Verification items for the finished model (mm, model axes). A direction names the side the tool comes from. Round coordinates to 2 decimals unless told otherwise and drop trailing zeros. Loops run counter-clockwise (first coordinate to the right, second up) from the corner with the lowest first, then second, coordinate; pieces in that order, holes last.
from build123d import *

# Parameters (mm, degrees)
SKETCH2_W          = 2.5
SKETCH2_H          = 3.5
CUT_EXTRUDE1_DEPTH = 3.5
FILLET1_R          = 0.5
CUT_EXTRUDE2_DEPTH = 0.5


with BuildPart() as part:
    # Sketch1 → Revolve1 (revolve)
    with BuildSketch(Plane.XY, mode=Mode.PRIVATE) as revolve1_sk:
        Polygon((0, 7.25), (5, 7.25), (5, 1.25), (8, 1.25), (8, 0), (0, 0), align=None)
    revolve(revolve1_sk.sketch.rotate(Axis((0, 7.25, 0), (0, -1, 0)), 180), axis=Axis((0, 7.25, 0), (0, -1, 0)))

    # Sketch2 → Cut-Extrude1 (cut)
    with BuildSketch(Plane.XZ):
        Rectangle(SKETCH2_W, SKETCH2_H)
    extrude(amount=-CUT_EXTRUDE1_DEPTH, mode=Mode.SUBTRACT)

    # Fillet1
    fillet1_edges = [part.edges().sort_by_distance(p)[0] for p in [
        (5, 7.25, 0),
    ]]
    fillet(fillet1_edges, radius=FILLET1_R)

    # Sketch3 → Cut-Extrude2 (cut)
    with BuildSketch(Plane(origin=(0, 7.25, 0), x_dir=(1, 0, 0), z_dir=(0, 1, 0))):
        Polygon((-2.230769231, 3), (-1.424278846, 3), (0.03125, 0.622596154), (1.486778846, 3), (2.307692308, 3), (0.466346154, 0.060096154), (2.384615385, -3), (1.563701923, -3), (0.03125, -0.503605769), (-1.501201923, -3), (-2.307692308, -3), (-0.389423077, 0.058894231), align=None)
    extrude(amount=-CUT_EXTRUDE2_DEPTH, mode=Mode.SUBTRACT)


solid = part.part
1. Tool access check on faces 5 (the face through (1.4, 7, -1.55)), 6 (the face through (-2, 0, 0)), 7 (the face through (-1.25, 2, 0)). Record the directions out of +Z, -Z, +X, -X, +Y, -Y that give a thin tool (end or side, any length) a straight path to the whole face; none if there is none.
2. Section check B-B (y = 4.25). Enter the section's corners in (x, z).
3. Section check C-C (x = -6.25). Enter the section's corners in (y, z), then the cut area to 3 significant figures.
4. Section check D-D (x = 5.75). Enter the section's corners in (y, z), then the cut area to 3 significant figures.
5. Scan lines: L1, parallel to Y at x = -1, z = 7; L2, parallel to X at y = 7, z = -0.25; L3, parallel to Z at x = 4, y = 6.75. Record each from-to range of solid material in increasing order.
6. Section check A-A (y = 1.75). Enter the section's corners in (x, z).
7. Gauge pin test, flat ends, axial feed: P1, Ø3, axis at x = 4.5, y = 4, coming from the -Z side; P2, Ø1.4, axis at x = 0, z = 0.5, coming from the +Y side; P3, Ø2, axis at y = 4, z = 2.5, coming from the -X side; P4, Ø3, axis at x = -1.5, y = 3, coming from the -Z side. Record the tip position at first contact, or that the pin passes through.
8. Release check for a two-part mould opening along Z. For faces 1 (the face through (1, 7.25, 0)), 2 (the face through (-1.36, 7, 1.49)), 3 (the face through (1.73, 0.62, 7.81)), 4 (the face through (0, 3.5, 0)) record: released by +Z, released by -Z, zero draft, split by the parting line, or undercut.
Taken from the geometry:
1. face 5: +Y
1. face 6: +Z, -Z, +X, -X, -Y
1. face 7: -Y
2. outline: circle Ø10 at (0, 0)
3. outline: (0, -4.99) - (1.25, -4.99) - (1.25, 4.99) - (0, 4.99) - close
3. area: 12.5 mm2
4. outline: (0, -5.56) - (1.25, -5.56) - (1.25, 5.56) - (0, 5.56) - close
4. area: 13.9 mm2
5. L1: y = 0 to 1.25
5. L2: x = -4.93 to -0.51, 0.59 to 4.93
5. L3: z = -3 to 3
6. outline: circle Ø10 at (0, 0); hole (-1.25, -1.75) - (1.25, -1.75) - (1.25, 1.75) - (-1.25, 1.75) - close
7. P1: stops at z = -4
7. P2: stops at y = 7.25
7. P3: stops at x = -4.77
7. P4: stops at z = -5
8. face 1: zero draft
8. face 2: undercut
8. face 3: split by the parting line
8. face 4: undercut
